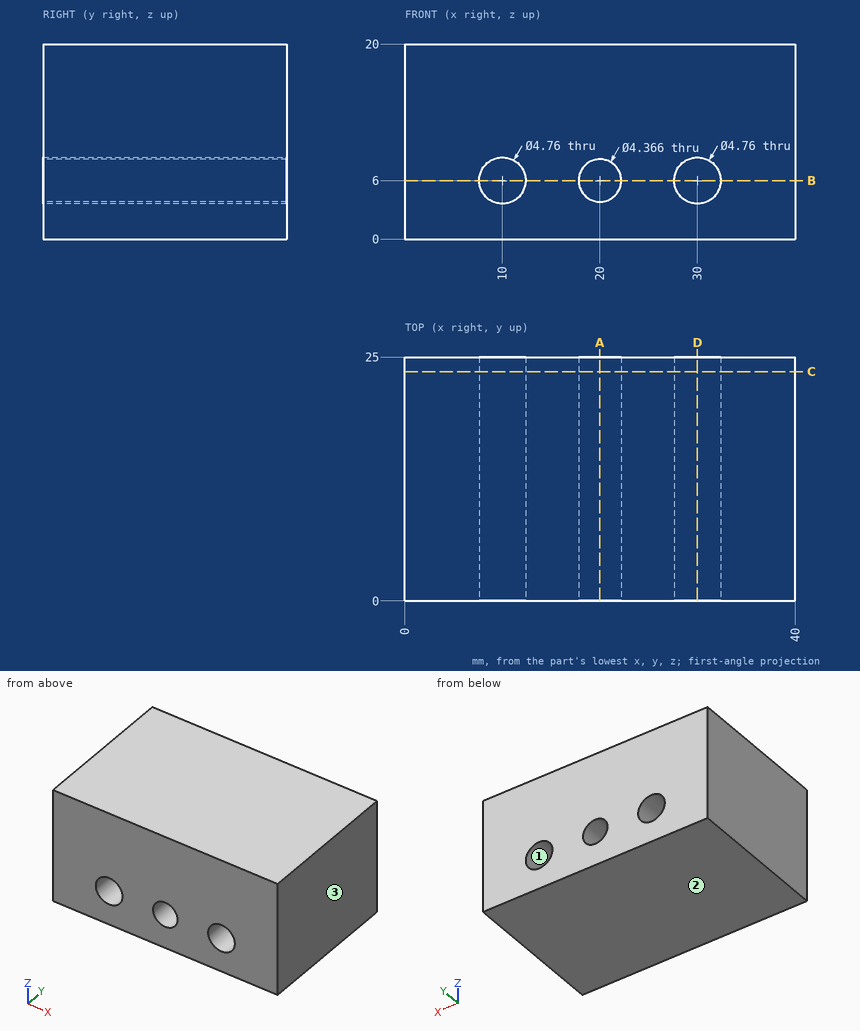
Job drawing, mm, ordinate dimensions from the low corner. One solid piece. Coordinates: 2 decimals unless noted, no trailing zeros. Write each loop counter-clockwise with the first axis right and the second up, starting at its lowest first coordinate (ties: lowest second). Pieces come first, ordered by that corner, then holes. Notation, with made-up numbers: (65.5, -9.5) - (80.5, -9.5) arc R16 ccw to (80.5, 8.5) - close; hole circle Ø9 at (-13.75, 32.25). An arc over 180 degrees is marked (long way). Use a Markdown table: item, result. Add a question column.
Item 1: Band-saw the part on D-D, the plane x = 30. Give the cut face in (y, z), and give its area (3 significant figures).
Item 2: Band-saw the part on B-B, the plane z = 6. Give the cut face in (x, y), and give its area (3 significant figures).
Item 3: Drill centre lines: L1, parallel to X at y = 11, z = 6; L2, parallel to X at y = 13, z = 4.5 (1 decimal); L3, parallel to Z at x = 20, y = 9.25. Where is each one in solid material? Low to high. Write a range as from..to.
Item 4: Flat gauge pin, fed straight in: pin 1 (8 mm diameter, centred on x = 34, z = 11.5, fed in from -Y). Where does the tip first touch, or does it go through?
Item 5: Mould opens along Z. For the marked faces 1, 2 and 3 say: pulls with the +Z half, pulls with the -Z half, needs draft (parallel to the pull), parting line crosses it, or undercut.
Item 6: Band-saw the part on C-C, the plane y = 23.5. Give the cut face in (x, z).
Item 7: Band-saw the part on A-A, the plane x = 20. Give the cut face in (y, z), and give its area (3 significant figures).
Numbers:
| question | item | result |
|---|---|---|
| 1 | outline | (0, 0) - (25, 0) - (25, 3.62) - (0, 3.62) - close; (0, 8.38) - (25, 8.38) - (25, 20) - (0, 20) - close |
| 1 | area | 381 mm2 |
| 2 | outline | (0, 0) - (7.62, 0) - (7.62, 25) - (0, 25) - close; (12.38, 0) - (17.82, 0) - (17.82, 25) - (12.38, 25) - close; (22.18, 0) - (27.62, 0) - (27.62, 25) - (22.18, 25) - close; (32.38, 0) - (40, 0) - (40, 25) - (32.38, 25) - close |
| 2 | area | 653 mm2 |
| 3 | L1 | 0..7.62, 12.38..17.82, 22.18..27.62, 32.38..40 |
| 3 | L2 | 0..8.2, 11.8..18.4, 21.6..28.2, 31.8..40 |
| 3 | L3 | 0..3.82, 8.18..20 |
| 4 | pin 1 | y = 0 |
| 5 | face 1 | undercut |
| 5 | face 2 | pulls with the -Z half |
| 5 | face 3 | needs draft |
| 6 | outline | (0, 0) - (40, 0) - (40, 20) - (0, 20) - close; hole circle Ø4.76 at (10, 6); hole circle Ø4.37 at (20, 6); hole circle Ø4.76 at (30, 6) |
| 7 | outline | (0, 0) - (25, 0) - (25, 3.82) - (0, 3.82) - close; (0, 8.18) - (25, 8.18) - (25, 20) - (0, 20) - close |
| 7 | area | 391 mm2 |
